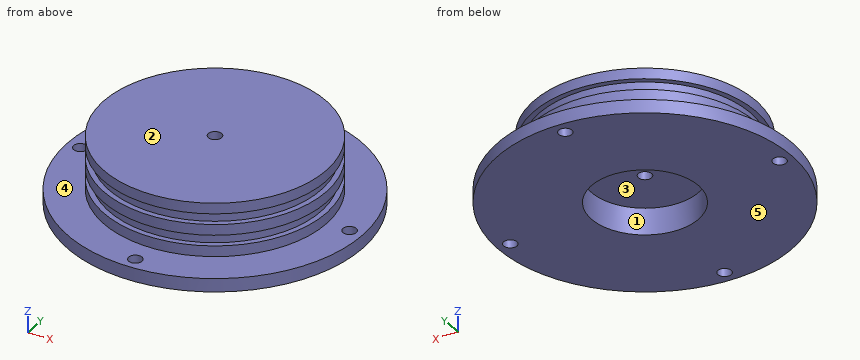
```python
from build123d import *

# Parameters (mm, degrees)
SKETCH1_R           = 55
BOSS_EXTRUDE1_DEPTH = 5
SKETCH3_R           = 2.5
CUT_EXTRUDE1_DEPTH  = 78.942286341
CIRPATTERN1_COUNT   = 4
SKETCH2_R           = 41.5
BOSS_EXTRUDE2_DEPTH = 20
SKETCH4_W           = 4
SKETCH4_H           = 2
SKETCH5_R           = 2.5
CUT_EXTRUDE2_DEPTH  = 82.700673192
SKETCH6_R           = 20
CUT_EXTRUDE3_DEPTH  = 10


with BuildPart() as part:
    # Sketch1 → Boss-Extrude1 (new body)
    with BuildSketch(Plane.XY):
        Circle(SKETCH1_R)
    extrude(amount=BOSS_EXTRUDE1_DEPTH)

    # Sketch3 → Cut-Extrude1 (cut, through all)
    with BuildSketch(Plane(origin=(0, 0, 0), x_dir=(-1, 0, 0), z_dir=(0, 0, -1))):
        with Locations((0, 50)):
            Circle(SKETCH3_R)
    cut_extrude1 = extrude(amount=-CUT_EXTRUDE1_DEPTH, mode=Mode.SUBTRACT)

    # CirPattern1: Cut-Extrude1 ×4 about axis
    cirpattern1_axis = Axis((0, 0, 0), (0, 0, 1))
    for i in range(1, CIRPATTERN1_COUNT):
        add(cut_extrude1.rotate(cirpattern1_axis, i * 360 / CIRPATTERN1_COUNT), mode=Mode.SUBTRACT)

    # Sketch2 → Boss-Extrude2 (add)
    with BuildSketch(Plane.XY.offset(5)):
        Circle(SKETCH2_R)
    extrude(amount=BOSS_EXTRUDE2_DEPTH)

    # Sketch4 → Cut-Revolve1 (revolve, cut)
    with BuildSketch(Plane(origin=(0, 0, 0), x_dir=(0, 0, -1), z_dir=(1, 0, 0))):
        with Locations((-11, 40.5)):
            Rectangle(SKETCH4_W, SKETCH4_H)
        with Locations((-19, 40.5)):
            Rectangle(SKETCH4_W, SKETCH4_H)
    revolve(axis=Axis((0, 0, 0), (0, 0, 1)), mode=Mode.SUBTRACT)

    # Sketch5 → Cut-Extrude2 (cut, through all)
    with BuildSketch(Plane(origin=(0, 0, 0), x_dir=(-1, 0, 0), z_dir=(0, 0, -1))):
        Circle(SKETCH5_R)
    extrude(amount=-CUT_EXTRUDE2_DEPTH, mode=Mode.SUBTRACT)

    # Sketch6 → Cut-Extrude3 (cut)
    with BuildSketch(Plane(origin=(0, 0, 0), x_dir=(-1, 0, 0), z_dir=(0, 0, -1))):
        Circle(SKETCH6_R)
    extrude(amount=-CUT_EXTRUDE3_DEPTH, mode=Mode.SUBTRACT)


solid = part.part
```
For this review, take the finished solid that the model builds, in its own axes (mm). Face numbers are marked on the shaded views. A direction names the side the tool comes from. Round coordinates to 2 decimals unless told otherwise and drop trailing zeros. Write each loop counter-clockwise with the first axis right and the second up, starting at its lowest first coordinate (ties: lowest second). Pieces come first, ordered by that corner, then holes. Notation, with made-up numbers: (25, 60) -> (46, 60) arc R19 ccw to (46, 68) -> close; hole circle Ø8 at (18, 89). An arc over 180 degrees is marked (long way). One line per question, with ' | ' between items. Start each with the question number.
1) For pin 1 Ø25 at (x, y) = (-12, 4) entering from -Z; pin 2 Ø4 at (x, y) = (50, 0) entering from -Z; pin 3 Ø10 at (x, z) = (-17, 2.5) entering from +Y; pin 4 Ø6 at (x, y) = (0, -50) entering from +Z, all flat-tipped, find the tip position at first contact; note any pin that passes through.
2) Mouldability with a two-part tool opening along X and no side actions: class the marked faces 1 and 2 as +X half, -X half, draft (parallel to the pull), parting line (faces both ways), or undercut.
3) Add section B-B (y = 0). Count the separate pieces of the cut face and the enclosed holes in it, and give its area (3 significant figures).
4) Add section D-D (y = -32). Write out the cut boundary in (x, z), and give its area (3 significant figures).
5) Wall thickness on line 1 along Z through (x, y) = (-23.5, -33.5); line 2 along Y through (x, z) = (0, 5.25); line 3 along Z through (x, y) = (45, 21): over which ranges is each line inside the solid? List them lowest first.
6) Add section A-A (x = 50). Write out the cut boundary in (y, z), and give its area (3 significant figures).
7) Machinability: for the marked faces 3, 4 and 5, which of the approach directions +Z, -Z, +X, -X, +Y, -Y give a long, thin tool a straight path to every point of the face, cutting with its end or side? Answer none if there is none.
Reported:
1) pin 1: stops at z = 0 | pin 2: passes through | pin 3: stops at y = 53.67 | pin 4: stops at z = 5
2) face 1: undercut | face 2: draft
3) separate pieces: 4 | enclosed holes: 0 | area: 1,650 mm²
4) outline: (-44.73, 0) -> (44.73, 0) -> (44.73, 5) -> (26.42, 5) -> (26.42, 9) -> (23.16, 9) -> (23.16, 13) -> (26.42, 13) -> (26.42, 17) -> (23.16, 17) -> (23.16, 21) -> (26.42, 21) -> (26.42, 25) -> (-26.42, 25) -> (-26.42, 21) -> (-23.16, 21) -> (-23.16, 17) -> (-26.42, 17) -> (-26.42, 13) -> (-23.16, 13) -> (-23.16, 9) -> (-26.42, 9) -> (-26.42, 5) -> (-44.73, 5) -> close | area: 1,450 mm²
5) line 1: z = 0 to 9, 13 to 17, 21 to 25 | line 2: y = -41.5 to -20, 20 to 41.5 | line 3: z = 0 to 5
6) outline: (-22.91, 0) -> (-2.5, 0) -> (-2.5, 5) -> (-22.91, 5) -> close; (2.5, 0) -> (22.91, 0) -> (22.91, 5) -> (2.5, 5) -> close | area: 204 mm²
7) face 3: -Z | face 4: +Z | face 5: -Z, +X, -X, +Y, -Y
